```python
from build123d import *

# Parameters (mm, degrees)
SKETCH1_R                                         = 14
SKETCH1_R_2                                       = 4
SKETCH1_R_3                                       = 1.5
BOSS_EXTRUDE1_DEPTH                               = 5
CUT_EXTRUDE4_START                                = -3
CUT_EXTRUDE4_DEPTH                                = 3
SKETCH14_R                                        = 13.5
CUT_EXTRUDE5_DEPTH                                = 2
FILLET2_R                                         = 1
BOSS_EXTRUDE2_DEPTH                               = 1
BOSS_EXTRUDE2_DEPTH_BACK                          = 3
SKETCH16_R                                        = 1.5
BOSS_EXTRUDE4_DEPTH                               = 1
BOSS_EXTRUDE4_DEPTH_BACK                          = 3
SKETCH17_R                                        = 1.5
SKETCH17_R_2                                      = 1.550441812
SKETCH17_R_3                                      = 1.546716968
CSK_FOR_M2_5_FLAT_HEAD_MACHINE_SCREW1_D           = 2.7
CSK_FOR_M2_5_FLAT_HEAD_MACHINE_SCREW1_CSINK_D     = 5.5
CSK_FOR_M2_5_FLAT_HEAD_MACHINE_SCREW1_CSINK_ANGLE = 90
CSK_FOR_M2_5_FLAT_HEAD_MACHINE_SCREW2_D           = 2.7
CSK_FOR_M2_5_FLAT_HEAD_MACHINE_SCREW2_CSINK_D     = 5.5
CSK_FOR_M2_5_FLAT_HEAD_MACHINE_SCREW2_CSINK_ANGLE = 90
CSK_FOR_M2_5_FLAT_HEAD_MACHINE_SCREW3_D           = 2.7
CSK_FOR_M2_5_FLAT_HEAD_MACHINE_SCREW3_CSINK_D     = 5.5
CSK_FOR_M2_5_FLAT_HEAD_MACHINE_SCREW3_CSINK_ANGLE = 90
CSK_FOR_M2_5_FLAT_HEAD_MACHINE_SCREW4_D           = 2.7
CSK_FOR_M2_5_FLAT_HEAD_MACHINE_SCREW4_CSINK_D     = 5.5
CSK_FOR_M2_5_FLAT_HEAD_MACHINE_SCREW4_CSINK_ANGLE = 90
FILLET3_R                                         = 0.15


with BuildPart() as part:
    # Sketch1 → Boss-Extrude1 (new body)
    with BuildSketch(Plane.XY):
        Circle(SKETCH1_R)
        Circle(SKETCH1_R_2, mode=Mode.SUBTRACT)
        with Locations((-5.656854249, -5.656854249)):
            Circle(SKETCH1_R_3, mode=Mode.SUBTRACT)
        with Locations((5.656854249, 5.656854249)):
            Circle(SKETCH1_R_3, mode=Mode.SUBTRACT)
        with Locations((6.717514421, -6.717514421)):
            Circle(SKETCH1_R_3, mode=Mode.SUBTRACT)
        with Locations((-6.717514421, 6.717514421)):
            Circle(SKETCH1_R_3, mode=Mode.SUBTRACT)
    extrude(amount=BOSS_EXTRUDE1_DEPTH)

    # Sketch13 → Cut-Extrude4 (cut)
    with BuildSketch(Plane.XY.offset(5).offset(CUT_EXTRUDE4_START)):
        with BuildLine():
            Line((-11, 4), (-13.416407865, 4))
            ThreePointArc((-13.416407865, 4), (-14, 0), (-13.416407865, -4))
            Line((-13.416407865, -4), (-11, -4))
            ThreePointArc((-11, -4), (-7, 0), (-11, 4))
        make_face()
        with BuildLine():
            Line((4, 11), (4, 13.416407865))
            ThreePointArc((4, 13.416407865), (0, 14), (-4, 13.416407865))
            Line((-4, 13.416407865), (-4, 11))
            ThreePointArc((-4, 11), (0, 7), (4, 11))
        make_face()
        with BuildLine():
            Line((11, -4), (13.416407865, -4))
            ThreePointArc((13.416407865, -4), (14, 0), (13.416407865, 4))
            Line((13.416407865, 4), (11, 4))
            ThreePointArc((11, 4), (7, 0), (11, -4))
        make_face()
        with BuildLine():
            Line((-4, -11), (-4, -13.416407865))
            ThreePointArc((-4, -13.416407865), (0, -14), (4, -13.416407865))
            Line((4, -13.416407865), (4, -11))
            ThreePointArc((4, -11), (0, -7), (-4, -11))
        make_face()
    extrude(amount=CUT_EXTRUDE4_DEPTH, mode=Mode.SUBTRACT)

    # Sketch14 → Cut-Extrude5 (cut)
    with BuildSketch(Plane(origin=(0, 0, 0), x_dir=(-1, 0, 0), z_dir=(0, 0, -1))):
        Circle(SKETCH14_R)
    extrude(amount=-CUT_EXTRUDE5_DEPTH, mode=Mode.SUBTRACT)

    # Fillet2
    fillet2_edges = [part.edges().sort_by_distance(p)[0] for p in [
        (-9.899494937, -9.899494937, 5),
        (-9.899494937, 9.899494937, 5),
        (9.899494937, 9.899494937, 5),
        (9.899494937, -9.899494937, 5),
    ]]
    fillet(fillet2_edges, radius=FILLET2_R)

    # Sketch16 → Boss-Extrude2 (add, two sides: drawn at the far end of the back side and taken through both)
    with BuildSketch(Plane(origin=(0, 0, 2), x_dir=(-1, 0, 0), z_dir=(0, 0, -1)).offset(-BOSS_EXTRUDE2_DEPTH_BACK)):
        with Locations((6.717514421, 6.717514421)):
            Circle(SKETCH16_R)
    extrude(amount=BOSS_EXTRUDE2_DEPTH + BOSS_EXTRUDE2_DEPTH_BACK)

    # Sketch17 → Boss-Extrude4 (add, two sides: drawn at the far end of the back side and taken through both)
    with BuildSketch(Plane(origin=(0, 0, 2), x_dir=(-1, 0, 0), z_dir=(0, 0, -1)).offset(-BOSS_EXTRUDE4_DEPTH_BACK)):
        with Locations((-5.656854249, 5.656854249)):
            Circle(SKETCH17_R)
        with Locations((5.704995791, -5.671913081)):
            Circle(SKETCH17_R_2)
        with Locations((-6.763543143, -6.725503911)):
            Circle(SKETCH17_R_3)
    extrude(amount=BOSS_EXTRUDE4_DEPTH + BOSS_EXTRUDE4_DEPTH_BACK)

    # CSK for M2.5 Flat Head Machine Screw1 (through all)
    with Locations(Plane(origin=(-6.717514421, 6.717514421, 1), x_dir=(-1, 0, 0), z_dir=(0, 0, -1))):
        with Locations((0, 0)):
            CounterSinkHole(CSK_FOR_M2_5_FLAT_HEAD_MACHINE_SCREW1_D / 2, CSK_FOR_M2_5_FLAT_HEAD_MACHINE_SCREW1_CSINK_D / 2, counter_sink_angle=CSK_FOR_M2_5_FLAT_HEAD_MACHINE_SCREW1_CSINK_ANGLE)

    # CSK for M2.5 Flat Head Machine Screw2 (through all)
    with Locations(Plane(origin=(5.656854249, 5.656854249, 1), x_dir=(-1, 0, 0), z_dir=(0, 0, -1))):
        with Locations((0, 0)):
            CounterSinkHole(CSK_FOR_M2_5_FLAT_HEAD_MACHINE_SCREW2_D / 2, CSK_FOR_M2_5_FLAT_HEAD_MACHINE_SCREW2_CSINK_D / 2, counter_sink_angle=CSK_FOR_M2_5_FLAT_HEAD_MACHINE_SCREW2_CSINK_ANGLE)

    # CSK for M2.5 Flat Head Machine Screw3 (through all)
    with Locations(Plane(origin=(6.763543143, -6.725503911, 1), x_dir=(-1, 0, 0), z_dir=(0, 0, -1))):
        with Locations((0, 0)):
            CounterSinkHole(CSK_FOR_M2_5_FLAT_HEAD_MACHINE_SCREW3_D / 2, CSK_FOR_M2_5_FLAT_HEAD_MACHINE_SCREW3_CSINK_D / 2, counter_sink_angle=CSK_FOR_M2_5_FLAT_HEAD_MACHINE_SCREW3_CSINK_ANGLE)

    # CSK for M2.5 Flat Head Machine Screw4 (through all)
    with Locations(Plane(origin=(-5.704995791, -5.671913081, 1), x_dir=(-1, 0, 0), z_dir=(0, 0, -1))):
        with Locations((0, 0)):
            CounterSinkHole(CSK_FOR_M2_5_FLAT_HEAD_MACHINE_SCREW4_D / 2, CSK_FOR_M2_5_FLAT_HEAD_MACHINE_SCREW4_CSINK_D / 2, counter_sink_angle=CSK_FOR_M2_5_FLAT_HEAD_MACHINE_SCREW4_CSINK_ANGLE)

    # Fillet3
    fillet3_edges = [part.edges().sort_by_distance(p)[0] for p in [
        (-8.067514421, 6.717514421, 5),
        (4.306854249, 5.656854249, 5),
        (5.413543143, -6.725503911, 5),
        (-7.054995791, -5.671913081, 5),
    ]]
    fillet(fillet3_edges, radius=FILLET3_R)


solid = part.part
```
The listing builds one solid part. Answer for the finished solid, in the listing's coordinates (mm). A direction names the side the tool comes from. Give positions to 0.01 mm unless a question says otherwise; leave off trailing zeros. Order: outer loops, then holes, each group sorted by start corner. A loop starts at its lowest first (then second) coordinate and runs counter-clockwise, first axis right, second up. Notation, with made-up numbers: (40, 45) -> (78, 45) arc R12 cw to (78, 54) -> close; hole circle Ø11 at (6, -40). An arc over 180 degrees is marked (long way). Answer as a JSON object with one key per item and string values. Group by question number.
Item 1: Determine the mould class of faces 5 (the flat face through (-13.7, 0.1, 2)), 6 (the cylindrical face through (12.932, -5.362, 1.972)), 7 (the flat face through (-0.1, -13.7, 2)) for opening direction Y: pulls with the +Y half, pulls with the -Y half, needs draft (parallel to the pull), parting line crosses it, or undercut.
Item 2: The part is cut by section A-A on y = 0. Write down the section's boundary in (x, z).
Item 3: Flat-ended cylindrical pins translate along their axes: pin 1 (0.7 mm diameter, centred on y = 11.5, z = 3, fed in from +X); pin 2 (3 mm diameter, centred on y = -3.5, z = 4.5, fed in from -X); pin 3 (3 mm diameter, centred on x = 6.76, y = -6.73, fed in from -Z). Find the tip coordinate at first contact, or state that the pin passes through.
Item 4: The part is cut by section B-B on x = -1.25. Write down the section's boundary in (y, z), and give its area (3 significant figures).
Item 5: A tool of negligible diameter and unlimited length cuts with its end or side. For faces 1 (the flat face through (-12, -4, 3)), 2 (the flat face through (12, 4, 3)), 3 (the cylindrical face through (-7, 0, 3)), 4 (the flat face through (-4, 12, 3)), from which of +Z, -Z, +X, -X, +Y, -Y can it reach the whole face along a straight path? Write none if from no direction.
Item 6: Consider L1, parallel to Y at x = 0, z = 1.45; L2, parallel to Z at x = -7.5, y = 4.5. Determine where each line is inside the solid, lowest interval first. Write a range as from..to.
Item 7: The part is cut by section D-D on y = -6. Give the number of separate pieces and of enclosed holes in the cut face, and give its area (3 significant figures).
Item 8: The part is cut by section C-C on z = 0.55. Write down the section's boundary in (x, y), and give its area (3 significant figures).
Result set:
{
 "1": {"face 5": "undercut", "face 6": "parting line crosses it", "face 7": "needs draft"},
 "2": {"outline": "(-14, 0) -> (-13.5, 0) -> (-13.5, 2) -> (-14, 2) -> close; (-7, 2) -> (-4, 2) -> (-4, 5) -> (-7, 5) -> close; (4, 2) -> (7, 2) -> (7, 5) -> (4, 5) -> close; (13.5, 0) -> (14, 0) -> (14, 2) -> (13.5, 2) -> close"},
 "3": {"pin 1": "x = 8.47", "pin 2": "x = -13.42", "pin 3": "z = 2.24"},
 "4": {"outline": "(-13.94, 0) -> (-13.44, 0) -> (-13.44, 2) -> (-13.94, 2) -> close; (-7.2, 2) -> (-3.8, 2) -> (-3.8, 5) -> (-7.2, 5) -> close; (3.8, 2) -> (7.2, 2) -> (7.2, 5) -> (3.8, 5) -> close; (13.44, 0) -> (13.94, 0) -> (13.94, 2) -> (13.44, 2) -> close", "area": "22.4 mm²"},
 "5": {"face 1": "+Z, -X", "face 2": "+Z, +X", "face 3": "+Z, -Z, -X", "face 4": "+Z, +Y"},
 "6": {"L1": "-14..-13.5, 13.5..14", "L2": "2..5"},
 "7": {"separate pieces": "3", "enclosed holes": "0", "area": "62.6 mm²"},
 "8": {"outline": "circle Ø28 at (0, 0); hole circle Ø27 at (0, 0)", "area": "43.2 mm²"}
}
